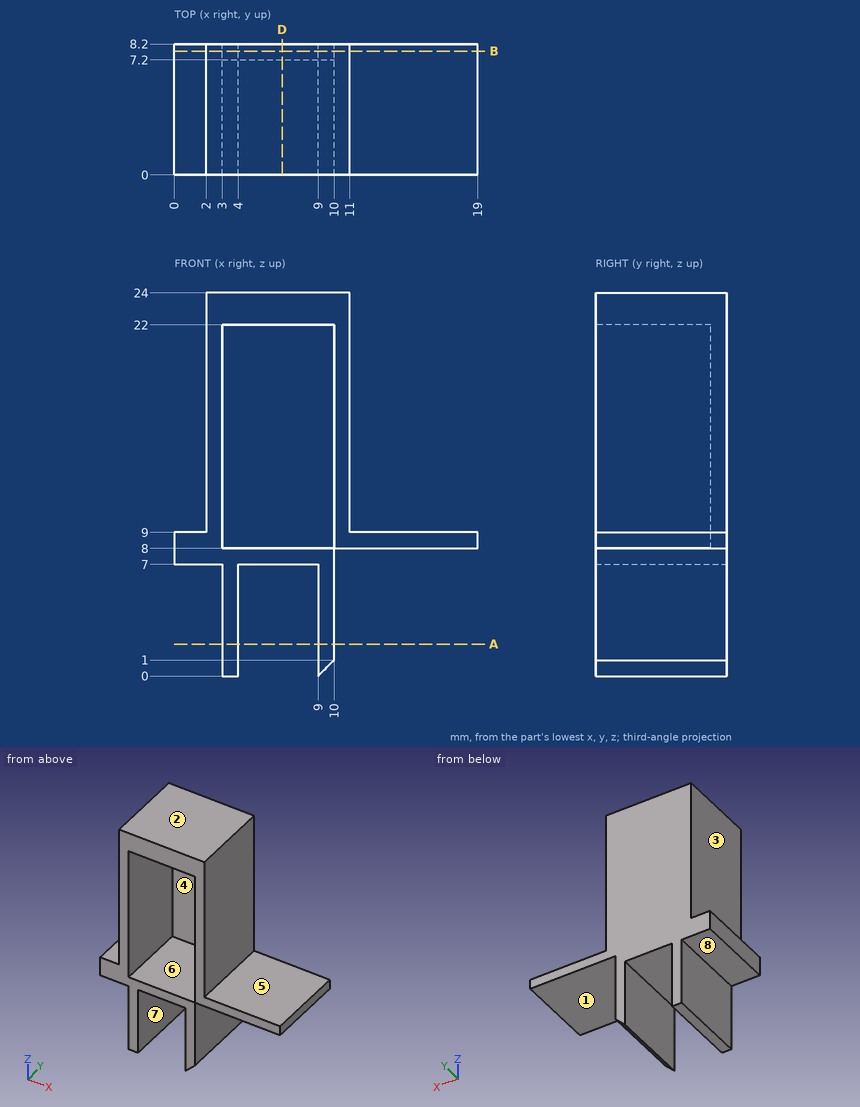
Check sheet for the drawn part. Datum: minimum x, y, z corner. Units: mm. A direction names the side the tool comes from. Give positions to 0.01 mm unless a question says otherwise; leave off trailing zeros. Order: outer loops, then holes, each group sorted by start corner. A loop starts at its lowest first (then second) coordinate and runs counter-clockwise, first axis right, second up. Notation, with made-up numbers: (10, -40) -> (60, -40) arc R14 cw to (60, -30) -> close; hole circle Ø6 at (64, 43). An arc over 180 degrees is marked (long way). Use a Markdown table: item, result.
1) Section check A-A, the plane z = 2. Record the boundary of the cut face in (x, y).
Results:
| item | result |
|---|---|
| outline | (3, 0) -> (4, 0) -> (4, 8.2) -> (3, 8.2) -> close; (9, 0) -> (10, 0) -> (10, 8.2) -> (9, 8.2) -> close |
2) Section check D-D, the plane x = 6.75. Record the boundary of the cut face in (y, z).
Results:
| item | result |
|---|---|
| outline | (0, 7) -> (8.2, 7) -> (8.2, 24) -> (0, 24) -> (0, 22) -> (7.2, 22) -> (7.2, 8) -> (0, 8) -> close |
3) Material ranges on probe 1 along X at (y, z) = (3, 17.25); probe 2 along Z at (x, y) = (5.5, 3.25); probe 3 along Z at (x, y) = (3.5, 6), recorded low to high.
Results:
| item | result |
|---|---|
| probe 1 | 2 to 3, 10 to 11 |
| probe 2 | 7 to 8, 22 to 24 |
| probe 3 | 0 to 8, 22 to 24 |
4) Tool access check on the marked faces 5, 6, 7 and 8. Record the directions out of +Z, -Z, +X, -X, +Y, -Y that give a thin tool (end or side, any length) a straight path to the whole face; none if there is none.
Results:
| item | result |
|---|---|
| face 5 | +Z, +X, +Y, -Y |
| face 6 | -Y |
| face 7 | -Z, +Y, -Y |
| face 8 | -Z, -X, +Y, -Y |
5) Mould release check, pull along Z, two halves, no side actions. Record for the marked faces 1, 2, 3 and 4: pulls with the +Z half, pulls with the -Z half, needs draft (parallel to the pull), parting line crosses it, or undercut.
Results:
| item | result |
|---|---|
| face 1 | pulls with the -Z half |
| face 2 | pulls with the +Z half |
| face 3 | needs draft |
| face 4 | undercut |
6) Depth check by flat-ended pin: pin 1 Ø2.5 at (x, y) = (16, 2) entering from +Z; pin 2 Ø1 at (y, z) = (2.5, 15.5) entering from +X; pin 3 Ø2 at (x, y) = (6, 5.5) entering from -Z; pin 4 Ø4 at (x, z) = (15, 5) entering from -Y. Enter the tip coordinate at first touch or a pass-through.
Results:
| item | result |
|---|---|
| pin 1 | z = 9 |
| pin 2 | x = 11 |
| pin 3 | z = 7 |
| pin 4 | through |
7) Section check B-B, the plane y = 7.75. Record the boundary of the cut face in (x, z), then the cut area to 4 significant figures.
Results:
| item | result |
|---|---|
| outline | (0, 7) -> (3, 7) -> (3, 0) -> (4, 0) -> (4, 7) -> (9, 7) -> (9, 0) -> (10, 1) -> (10, 8) -> (19, 8) -> (19, 9) -> (11, 9) -> (11, 24) -> (2, 24) -> (2, 9) -> (0, 9) -> close |
| area | 177.5 mm² |
